CAD build for the part. Positions are in the model's coordinates, mm. Face numbers are marked on the shaded views. A direction names the side the tool comes from. Round coordinates to 2 decimals unless told otherwise and drop trailing zeros. Write each loop counter-clockwise with the first axis right and the second up, starting at its lowest first coordinate (ties: lowest second). Pieces come first, ordered by that corner, then holes. Notation, with made-up numbers: (70.5, 7.5) - (96.5, 7.5) arc R7 cw to (96.5, 17.5) - close; hole circle Ø4 at (24.5, -6). An arc over 180 degrees is marked (long way). Put each result on its own line as item: value. Start each with the question number.
Item 1: Pin check, flat tip, straight feed: pin 1 Ø5.5 at (x, z) = (123.825, -88.9) entering from +Y. Stop position of the tip, or through.
Item 2: Cut at C-C (x = 91.5). Give the cut face in (y, z), and give its area (3 significant figures).
Item 3: 3-axis set-ups, long thin cutter, end or side, ignore diameter. For the marked faces 1, 2 and 3: which of +Z, -Z, +X, -X, +Y, -Y reach the whole face in a straight line?
Item 4: Cut at A-A (z = -19.05). Give the cut face in (x, y), and give its area (3 significant figures).
Item 5: Mould opens along X. For the marked faces 4, 5, 6 and 7 say: released by +X, released by -X, zero draft, split by the parting line, or undercut.
Item 6: Cut at B-B (z = -80.5). Give the cut face in (x, y).
Item 7: Cut at D-D (y = 47). Give the cut face in (x, z).
Item 8: Drill centre lines: line 1 (X direction, y = -20, z = -52.5); line 2 (Y direction, x = 36, z = -47); line 3 (Z direction, x = 110.5, y = 59.5). Where is each one in solid material? Low to high. Write a range as from..to.
```python
from build123d import *

# Parameters (mm, degrees)
BASE_FLANGE2_DEPTH     = 2.3622
SKETCHED_START         = -95.25
SKETCHED_BEND2_DEPTH   = 107.95
SKETCHED_BEND2_2_DEPTH = 107.95
SKETCHED_START_2       = 38.1
SKETCHED_BEND3_DEPTH   = 107.95
SKETCHED_BEND3_2_DEPTH = 107.95
SKETCH15_R             = 3.175
SKETCH15_R_2           = 1.905
SKETCH15_R_3           = 1.55
CUT_EXTRUDE1_DEPTH     = 166.131598701
SKETCH16_R             = 2.38125
CUT_EXTRUDE2_DEPTH     = 197.530978228
CUT_EXTRUDE3_REACH     = 193.008
SKETCH18_R             = 2.38125
SKETCH18_R_2           = 1.79959


# Read off the part's stored shape, not the designer's step: Sketched Bend2, Sketched Bend3
# Sheet-metal steps are written as plain solids
with BuildPart() as part:
    # Sketch7 → Base-Flange2 (new body)
    with BuildSketch(Plane(origin=(0, 0, 0), x_dir=(1, 0, 0), z_dir=(0, 1, 0))):
        Polygon((38.1, 95.25), (38.1, 165.1), (146.05, 165.1), (146.05, 95.25), (184.15, 95.25), (184.15, -12.7), (0, -12.7), (0, 95.25), align=None)
    extrude(amount=-BASE_FLANGE2_DEPTH)

    # Sketched Bend2 outline → Sketched Bend2 (cut)
    with BuildSketch(Plane.XY.offset(SKETCHED_START)):
        with BuildLine():
            Line((0, -2.3622), (35.090019621, -2.3622))
            ThreePointArc((35.090019621, -2.3622), (36.186889266, -0.661061548), (38.1, 0))
            Line((38.1, 0), (0, 0))
            Line((0, 0), (0, -2.3622))
        make_face()
        with BuildLine():
            ThreePointArc((146.05, 0), (147.963110734, -0.661061548), (149.059980379, -2.3622))
            Line((149.059980379, -2.3622), (184.15, -2.3622))
            Line((184.15, -2.3622), (184.15, 0))
            Line((184.15, 0), (146.05, 0))
        make_face()
    extrude(amount=SKETCHED_BEND2_DEPTH, mode=Mode.SUBTRACT)

    # Sketched Bend2 2 outline → Sketched Bend2 2 (add)
    with BuildSketch(Plane.XY.offset(SKETCHED_START)):
        with BuildLine():
            Line((37.3634, -38.186483884), (37.3634, -3.0988))
            ThreePointArc((37.3634, -3.0988), (37.579145145, -2.577945145), (38.1, -2.3622))
            Line((38.1, -2.3622), (35.090019621, -2.3622))
            ThreePointArc((35.090019621, -2.3622), (35.023485037, -2.727832183), (35.0012, -3.0988))
            Line((35.0012, -3.0988), (35.0012, -38.186483884))
            Line((35.0012, -38.186483884), (37.3634, -38.186483884))
        make_face()
        with BuildLine():
            Line((149.059980379, -2.3622), (146.05, -2.3622))
            ThreePointArc((146.05, -2.3622), (146.570854855, -2.577945145), (146.7866, -3.0988))
            Line((146.7866, -3.0988), (146.7866, -38.186483884))
            Line((146.7866, -38.186483884), (149.1488, -38.186483884))
            Line((149.1488, -38.186483884), (149.1488, -3.0988))
            ThreePointArc((149.1488, -3.0988), (149.126514963, -2.727832183), (149.059980379, -2.3622))
        make_face()
    extrude(amount=SKETCHED_BEND2_2_DEPTH)

    # Sketched Bend3 outline → Sketched Bend3 (cut)
    with BuildSketch(Plane.YZ.offset(SKETCHED_START_2)):
        with BuildLine():
            ThreePointArc((0, -98.259980379), (-1.701138452, -97.163110734), (-2.3622, -95.25))
            Line((-2.3622, -95.25), (-2.3622, -165.1))
            Line((-2.3622, -165.1), (0, -165.1))
            Line((0, -165.1), (0, -98.259980379))
        make_face()
    extrude(amount=SKETCHED_BEND3_DEPTH, mode=Mode.SUBTRACT)

    # Sketched Bend3 2 outline → Sketched Bend3 2 (add)
    with BuildSketch(Plane.YZ.offset(SKETCHED_START_2)):
        with BuildLine():
            Line((0, -95.25), (0, -98.259980379))
            ThreePointArc((0, -98.259980379), (0.365632183, -98.326514963), (0.7366, -98.3488))
            Line((0.7366, -98.3488), (67.574283884, -98.3488))
            Line((67.574283884, -98.3488), (67.574283884, -95.9866))
            Line((67.574283884, -95.9866), (0.7366, -95.9866))
            ThreePointArc((0.7366, -95.9866), (0.215745145, -95.770854855), (0, -95.25))
        make_face()
    extrude(amount=SKETCHED_BEND3_2_DEPTH)

    # Sketch15 → Cut-Extrude1 (cut, through all)
    with BuildSketch(Plane(origin=(149.1488, 0, 0), x_dir=(0, 0, -1), z_dir=(1, 0, 0))):
        with Locations(Location((6.35, -25.486483884, 0), (0, 0, 90))):
            Circle(SKETCH15_R)
        with Locations(Location((19.05, -25.486483884, 0), (0, 0, 90))):
            Circle(SKETCH15_R_2)
        with Locations(Location((31.75, -25.486483884, 0), (0, 0, 90))):
            Circle(SKETCH15_R_2)
        with Locations(Location((-6.35, -25.486483884, 0), (0, 0, 90))):
            Circle(SKETCH15_R_2)
        with Locations(Location((87.75, -13.186483884, 0), (0, 0, 90))):
            Circle(SKETCH15_R_3)
        with Locations(Location((47.05, -29.486483884, 0), (0, 0, 90))):
            Circle(SKETCH15_R_3)
        with Locations(Location((87.75, -29.486483884, 0), (0, 0, 90))):
            Circle(SKETCH15_R_3)
        with Locations(Location((47.05, -13.186483884, 0), (0, 0, 90))):
            Circle(SKETCH15_R_3)
    extrude(amount=-CUT_EXTRUDE1_DEPTH, mode=Mode.SUBTRACT)

    # Sketch16 → Cut-Extrude2 (cut, through all)
    with BuildSketch(Plane.XY.offset(-95.9866)):
        with Locations((63.5, 61.224283884)):
            Circle(SKETCH16_R)
        with Locations((120.65, 61.224283884)):
            Circle(SKETCH16_R)
        with Locations((63.5, 13.4366)):
            Circle(SKETCH16_R)
        with Locations((120.65, 13.4366)):
            Circle(SKETCH16_R)
    extrude(amount=-CUT_EXTRUDE2_DEPTH, mode=Mode.SUBTRACT)

    # Sketch18 → Cut-Extrude3 (cut, up to next)
    with BuildSketch(Plane(origin=(0, 0, 0), x_dir=(1, 0, 0), z_dir=(0, 1, 0)), mode=Mode.PRIVATE) as cut_extrude3_sk1:
        with Locations(Location((60.325, 88.9, 0), (0, 0, 270))):
            Circle(SKETCH18_R)
    cut_extrude3_tool1 = extrude(cut_extrude3_sk1.sketch, amount=-CUT_EXTRUDE3_REACH, mode=Mode.PRIVATE) & part.part
    # Sketch18 → Cut-Extrude3 (cut, up to next)
    with BuildSketch(Plane(origin=(0, 0, 0), x_dir=(1, 0, 0), z_dir=(0, 1, 0)), mode=Mode.PRIVATE) as cut_extrude3_sk2:
        with Locations(Location((123.825, 88.9, 0), (0, 0, 270))):
            Circle(SKETCH18_R)
    cut_extrude3_tool2 = extrude(cut_extrude3_sk2.sketch, amount=-CUT_EXTRUDE3_REACH, mode=Mode.PRIVATE) & part.part
    # Sketch18 → Cut-Extrude3 (cut, up to next)
    with BuildSketch(Plane(origin=(0, 0, 0), x_dir=(1, 0, 0), z_dir=(0, 1, 0)), mode=Mode.PRIVATE) as cut_extrude3_sk3:
        with Locations(Location((60.325, 50.8, 0), (0, 0, 270))):
            Circle(SKETCH18_R)
    cut_extrude3_tool3 = extrude(cut_extrude3_sk3.sketch, amount=-CUT_EXTRUDE3_REACH, mode=Mode.PRIVATE) & part.part
    # Sketch18 → Cut-Extrude3 (cut, up to next)
    with BuildSketch(Plane(origin=(0, 0, 0), x_dir=(1, 0, 0), z_dir=(0, 1, 0)), mode=Mode.PRIVATE) as cut_extrude3_sk4:
        with Locations(Location((123.825, 50.8, 0), (0, 0, 270))):
            Circle(SKETCH18_R)
    cut_extrude3_tool4 = extrude(cut_extrude3_sk4.sketch, amount=-CUT_EXTRUDE3_REACH, mode=Mode.PRIVATE) & part.part
    # Sketch18 → Cut-Extrude3 (cut, up to next)
    with BuildSketch(Plane(origin=(0, 0, 0), x_dir=(1, 0, 0), z_dir=(0, 1, 0)), mode=Mode.PRIVATE) as cut_extrude3_sk5:
        with Locations(Location((60.09894, 34.86658, 0), (0, 0, 270))):
            Circle(SKETCH18_R_2)
    cut_extrude3_tool5 = extrude(cut_extrude3_sk5.sketch, amount=-CUT_EXTRUDE3_REACH, mode=Mode.PRIVATE) & part.part
    # Sketch18 → Cut-Extrude3 (cut, up to next)
    with BuildSketch(Plane(origin=(0, 0, 0), x_dir=(1, 0, 0), z_dir=(0, 1, 0)), mode=Mode.PRIVATE) as cut_extrude3_sk6:
        with Locations(Location((110.20552, 39.59352, 0), (0, 0, 270))):
            Circle(SKETCH18_R_2)
    cut_extrude3_tool6 = extrude(cut_extrude3_sk6.sketch, amount=-CUT_EXTRUDE3_REACH, mode=Mode.PRIVATE) & part.part
    # Sketch18 → Cut-Extrude3 (cut, up to next)
    with BuildSketch(Plane(origin=(0, 0, 0), x_dir=(1, 0, 0), z_dir=(0, 1, 0)), mode=Mode.PRIVATE) as cut_extrude3_sk7:
        with Locations(Location((110.8202, -6.35, 0), (0, 0, 270))):
            Circle(SKETCH18_R_2)
    cut_extrude3_tool7 = extrude(cut_extrude3_sk7.sketch, amount=-CUT_EXTRUDE3_REACH, mode=Mode.PRIVATE) & part.part
    add(cut_extrude3_tool1.solids().sort_by_distance((60.325, 0, -88.9))[0], mode=Mode.SUBTRACT)
    add(cut_extrude3_tool2.solids().sort_by_distance((123.825, 0, -88.9))[0], mode=Mode.SUBTRACT)
    add(cut_extrude3_tool3.solids().sort_by_distance((60.325, 0, -50.8))[0], mode=Mode.SUBTRACT)
    add(cut_extrude3_tool4.solids().sort_by_distance((123.825, 0, -50.8))[0], mode=Mode.SUBTRACT)
    add(cut_extrude3_tool5.solids().sort_by_distance((60.09894, 0, -34.86658))[0], mode=Mode.SUBTRACT)
    add(cut_extrude3_tool6.solids().sort_by_distance((110.20552, 0, -39.59352))[0], mode=Mode.SUBTRACT)
    add(cut_extrude3_tool7.solids().sort_by_distance((110.8202, 0, 6.35))[0], mode=Mode.SUBTRACT)


solid = part.part
```
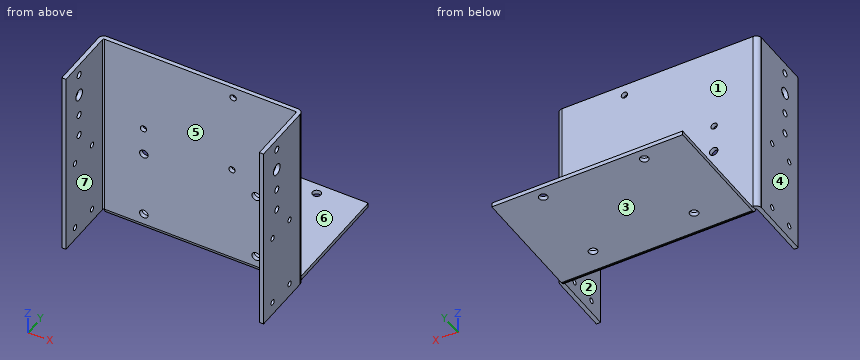
Output values:
1. pin 1: y = 0
2. outline: (-2.36, -95.25) arc R3.1 ccw to (0.74, -98.35) - (67.57, -98.35) - (67.57, -95.99) - (0.74, -95.99) arc R0.74 cw to (0, -95.25) - (0, 12.7) - (-2.36, 12.7) - close
2. area: 420 mm2
3. face 1: +Z, +X, -X, +Y
3. face 2: +Z, -Z, -Y
3. face 3: -Z, +X, -X, +Y, -Y
4. outline: (35, -38.19) - (37.36, -38.19) - (37.36, -27.39) - (35, -27.39) - close; (35, -23.58) - (37.36, -23.58) - (37.36, -3.1) arc R0.74 cw to (38.1, -2.36) - (146.05, -2.36) arc R0.74 cw to (146.79, -3.1) - (146.79, -23.58) - (149.15, -23.58) - (149.15, -3.1) arc R3.1 ccw to (146.05, 0) - (38.1, 0) arc R3.1 ccw to (35, -3.1) - close; (146.79, -38.19) - (149.15, -38.19) - (149.15, -27.39) - (146.79, -27.39) - close
4. area: 417 mm2
5. face 4: released by -X
5. face 5: undercut
5. face 6: zero draft
5. face 7: undercut
6. outline: (35, -38.19) - (37.36, -38.19) - (37.36, -3.1) arc R0.74 cw to (38.1, -2.36) - (146.05, -2.36) arc R0.74 cw to (146.79, -3.1) - (146.79, -38.19) - (149.15, -38.19) - (149.15, -3.1) arc R3.1 ccw to (146.05, 0) - (38.1, 0) arc R3.1 ccw to (35, -3.1) - close
7. outline: (38.1, -98.35) - (146.05, -98.35) - (146.05, -95.99) - (38.1, -95.99) - close
8. line 1: 35..37.36, 146.79..149.15
8. line 2: -38.19..-31.04, -27.94..-14.74, -11.64..-0.82
8. line 3: -98.35..-95.99
